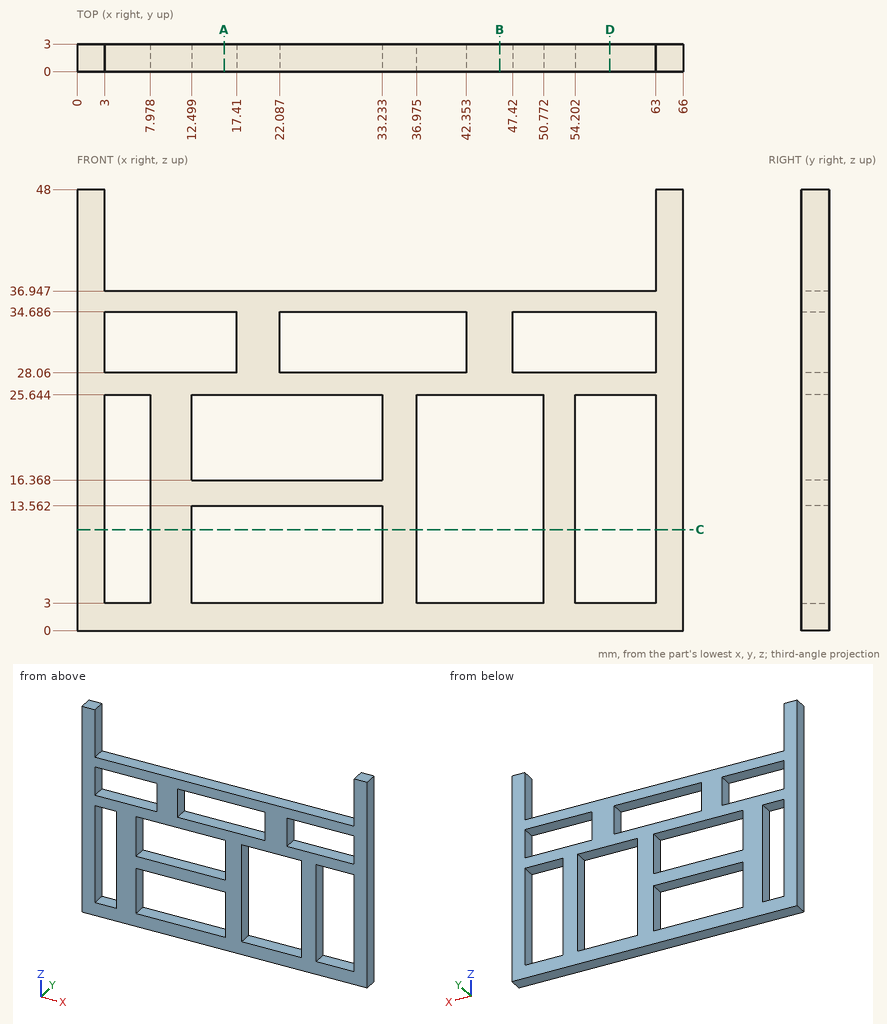
For this review, use the dimensioned drawing (mm, ordinates from the lowest corner) and the shaded views. Give positions to 0.01 mm unless a question says otherwise; leave off trailing zeros. Order: outer loops, then holes, each group sorted by start corner. A loop starts at its lowest first (then second) coordinate and runs counter-clockwise, first axis right, second up. Notation, with made-up numbers: M 31,13 L 86,13 A32 cw 86,46 Z; hole C 67,88 d1. An arc over 180 degrees is marked long. One line per question, with ' | ' between items. Start each with the question number.
1) Consider section C-C, the plane z = 11. Give the boundary of the cut face in (x, y) (1 decimal).
2) Consider section D-D, the plane x = 58. Give the boundary of the cut face in (y, z).
3) Wall thickness on L1, parallel to Z at x = 49, y = 1.9; L2, parallel to X at y = 0.35, z = 22.5 (1 decimal); L3, parallel to Z at x = 15.5, y = 1.5: over which ranges is each line inside the solid? List them lowest first. Write a range as from..to.
4) Consider section A-A, the plane x = 16. Give the boundary of the cut face in (y, z).
5) Consider section B-B, the plane x = 46. Give the boundary of the cut face in (y, z), then the cut area to 3 significant figures.
6) Clearance check with flat-ended pins moving along their axes: P1, Ø1.5, axis at x = 35, z = 14.5, coming from the -Y side; P2, Ø1, axis at x = 45.5, y = 0.5, coming from the +Z side. State where each tip first meets the part, or that it passes through.
Found:
1) outline: M 0,0 L 3,0 L 3,3 L 0,3 Z; M 8,0 L 12.5,0 L 12.5,3 L 8,3 Z; M 33.2,0 L 37,0 L 37,3 L 33.2,3 Z; M 50.8,0 L 54.2,0 L 54.2,3 L 50.8,3 Z; M 63,0 L 66,0 L 66,3 L 63,3 Z
2) outline: M 0,0 L 3,0 L 3,3 L 0,3 Z; M 0,25.64 L 3,25.64 L 3,28.06 L 0,28.06 Z; M 0,34.69 L 3,34.69 L 3,36.95 L 0,36.95 Z
3) L1: z = 0..3, 25.64..28.06, 34.69..36.95 | L2: x = 0..3, 8..12.5, 33.2..37, 50.8..54.2, 63..66 | L3: z = 0..3, 13.56..16.37, 25.64..28.06, 34.69..36.95
4) outline: M 0,0 L 3,0 L 3,3 L 0,3 Z; M 0,13.56 L 3,13.56 L 3,16.37 L 0,16.37 Z; M 0,25.64 L 3,25.64 L 3,28.06 L 0,28.06 Z; M 0,34.69 L 3,34.69 L 3,36.95 L 0,36.95 Z
5) outline: M 0,0 L 3,0 L 3,3 L 0,3 Z; M 0,25.64 L 3,25.64 L 3,36.95 L 0,36.95 Z | area: 42.9 mm²
6) P1: stops at y = 0 | P2: stops at z = 36.95
